Input: dimensioned drawing with shaded views. Units: mm. Origin: part minimum x, y, z. Give positions to 0.01 mm unless a question says otherwise; leave off trailing zeros. Loops run counter-clockwise (first coordinate to the right, second up) from the corner with the lowest first, then second, coordinate; pieces in that order, holes last.
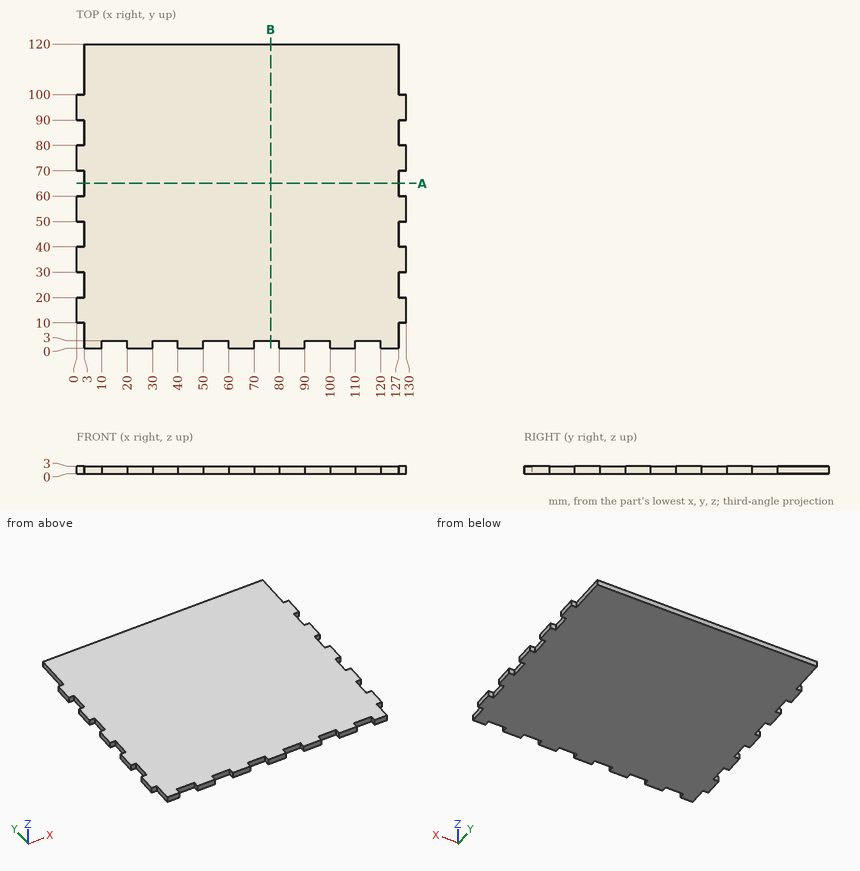
(1) First-contact query: pin 1 (0.9 mm diameter, centred on x = 113, z = 1, fed in from -Y); pin 2 (0.9 mm diameter, centred on x = 129, z = 1, fed in from -Y); pin 3 (0.9 mm diameter, centred on y = 1, z = 2, fed in from +X). Flat tips, straight axial feed; report the tip coordinate or a pass-through.
A:
pin 1: stops at y = 3
pin 2: stops at y = 10
pin 3: stops at x = 127
(2) Ray query, line 1 along Y through (x, z) = (56, 0.3); line 2 along X through (y, z) = (112.5, 1). Return the intervals inside material, ascending.
A:
line 1: y = 3 to 120
line 2: x = 3 to 127
(3) Section A-A, the plane y = 65. Return the cut outline in (x, z), then the cut area to 3 significant figures.
A:
outline: (3, 0) - (127, 0) - (127, 3) - (3, 3) - close
area: 372 mm2
(4) Section B-B, the plane x = 76.5. Return the cut outline in (y, z).
A:
outline: (3, 0) - (120, 0) - (120, 3) - (3, 3) - close
